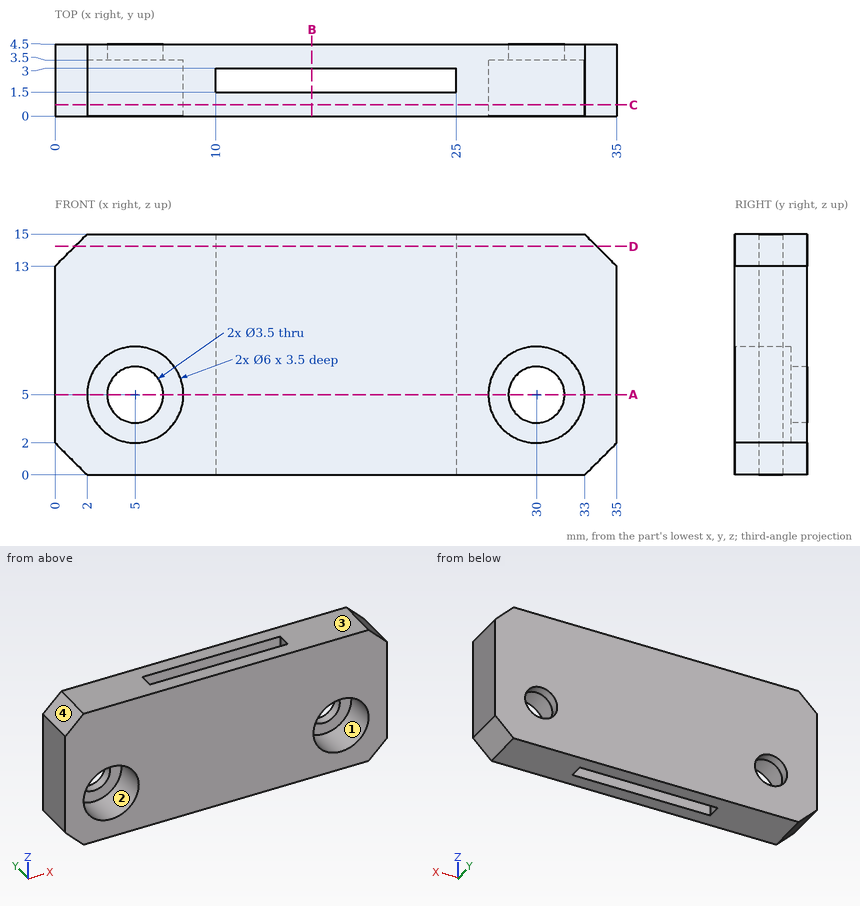
Geometry check sheet. Reference: drawing and pictorial views, mm from the part's lowest x, y, z. Round coordinates to 2 decimals unless told otherwise and drop trailing zeros. Write each loop counter-clockwise with the first axis right and the second up, starting at its lowest first coordinate (ties: lowest second). Pieces come first, ordered by that corner, then holes.
(1) Section check D-D (z = 14.25). Enter the section's corners in (x, y).
Returned:
outline: (1.25, 0) - (33.75, 0) - (33.75, 4.5) - (1.25, 4.5) - close; hole (10, 1.5) - (25, 1.5) - (25, 3) - (10, 3) - close
(2) Section check B-B (x = 16). Enter the section's corners in (y, z).
Returned:
outline: (0, 0) - (1.5, 0) - (1.5, 15) - (0, 15) - close; (3, 0) - (4.5, 0) - (4.5, 15) - (3, 15) - close
(3) Section check C-C (y = 0.7). Enter the section's corners in (x, z), plus the area to 3 significant figures.
Returned:
outline: (0, 2) - (2, 0) - (33, 0) - (35, 2) - (35, 13) - (33, 15) - (2, 15) - (0, 13) - close; hole circle Ø6 at (5, 5); hole circle Ø6 at (30, 5)
area: 460 mm2
(4) Section check A-A (z = 5). Enter the section's corners in (x, y), plus the area to 3 significant figures.
Returned:
outline: (0, 0) - (2, 0) - (2, 3.5) - (3.25, 3.5) - (3.25, 4.5) - (0, 4.5) - close; (6.75, 3.5) - (8, 3.5) - (8, 0) - (27, 0) - (27, 3.5) - (28.25, 3.5) - (28.25, 4.5) - (6.75, 4.5) - close; (31.75, 3.5) - (33, 3.5) - (33, 0) - (35, 0) - (35, 4.5) - (31.75, 4.5) - close; hole (10, 1.5) - (25, 1.5) - (25, 3) - (10, 3) - close
area: 86.0 mm2
(5) Material ranges on line 1 (X direction, y = 2.15, z = 5.25); line 2 (Y direction, x = 12, z = 1.5); line 3 (X direction, y = 1.8, z = 7.5), recorded low to high.
Returned:
line 1: x = 0 to 2.01, 7.99 to 10, 25 to 27.01, 32.99 to 35
line 2: y = 0 to 1.5, 3 to 4.5
line 3: x = 0 to 3.34, 6.66 to 10, 25 to 28.34, 31.66 to 35
(6) Mould release check, pull along X, two halves, no side actions. Record for the marked faces 1, 2, 3 and 4: pulls with the +X half, pulls with the -X half, needs draft (parallel to the pull), parting line crosses it, or undercut.
Returned:
face 1: undercut
face 2: undercut
face 3: needs draft
face 4: pulls with the -X half
(7) Depth check by flat-ended pin: pin 1 Ø1.8 at (x, z) = (3.5, 4.5) entering from -Y; pin 2 Ø2 at (x, z) = (5, 5) entering from +Y. Enter the tip coordinate at first touch or a pass-through.
Returned:
pin 1: stops at y = 3.5
pin 2: passes through
